Part model, mm, in its own coordinate system. A direction names the side the tool comes from. Give positions to 0.01 mm unless a question says otherwise; leave off trailing zeros. Order: outer loops, then holes, each group sorted by start corner. A loop starts at its lowest first (then second) coordinate and runs counter-clockwise, first axis right, second up.
1. Which spindle directions (+Z, -Z, +X, -X, +Y, -Y) get a long thin tool onto all of the face, cutting with end or side? Do faces 4 (the flat face through (19, -25, -8)), 5 (the cylindrical face through (4.17, 12.32, -18.8)), 6 (the flat face through (0, 25, 0)), 7 (the cylindrical face through (-15.201, -12.037, -11.655)). Say none if no direction does.
2. Drop flat-ended pins along their axis: pin 1 Ø1.5 at (y, z) = (-33, -12.5) entering from +X; pin 2 Ø8 at (x, y) = (-6.5, 8.5) entering from +Z; pin 3 Ø4 at (y, z) = (-23, 4.5) entering from -X. Give the stop position or say it passes through.
3. Mould opens along Z. For faces 1 (the cylindrical face through (20.445, -12.325, 6.438)), 2 (the flat face through (-11.2, 0, 16)), 3 (the cylindrical face through (-4.089, -12.04, -18.413)) say: +Z half, -Z half, draft (parallel to the pull), parting line (faces both ways), or undercut.
4. Slice it at C-C on y = -42.5. List the corners of the cut face in (x, z), and give its area (3 significant figures).
5. Probe line 1 (Z direction, x = 0, y = -12) (3 decimals); line 2 (X direction, y = -15, z = -1.5); line 3 (Z direction, x = 8, y = -9). List the from-to ranges inside material, lowest first.
6. Slice it at B-B on y = 14. List the corners of the cut face in (x, z), and give its area (3 significant figures).
7. Slice it at A-A on y = -11.5. List the corners of the cut face in (x, z) (3 decimals).
from build123d import *

# Parameters (mm, degrees)
F0_R     = 21.435
F0_R_2   = 19.35
F1_DEPTH = 25
F5_R     = 19.154771
F5_R_2   = 18.861777
F6_DEPTH = 25
F4_R     = 19.257792
F7_DEPTH = 25


with BuildPart() as f1:
    # F0 (on Front) → F1 (new body)
    with BuildSketch(Plane.XZ):
        Circle(F0_R)
        Circle(F0_R_2, mode=Mode.SUBTRACT)
    extrude(amount=F1_DEPTH)

    # F2 (on Right) → F3 (revolve)
    with BuildSketch(Plane.YZ):
        Polygon((-76.707862, 0), (-24.888575, 0), (-24.378041, 20.674003), align=None)
    revolve(axis=Axis((0, -6.062602, 0), (0, -1, 0)))

    # F5 (on Front) → F6 (join)
    with BuildSketch(Plane.XZ):
        Circle(F5_R)
        Circle(F5_R_2, mode=Mode.SUBTRACT)
    extrude(amount=F6_DEPTH)

    # F4 (on face) → F7 (join)
    with BuildSketch(Plane(origin=(0, 0, 0), x_dir=(-1, 0, 0), z_dir=(0, 1, 0))):
        Circle(F4_R)
    extrude(amount=F7_DEPTH)


solid = f1.part
Data:
1. face 4: -Y
1. face 5: +Y
1. face 6: +Z, -Z, +X, -X, +Y
1. face 7: none
2. pin 1: stops at x = 12.76
2. pin 2: stops at z = 19.09
2. pin 3: stops at x = -21.29
3. face 1: parting line
3. face 2: draft
3. face 3: undercut
4. outline: circle Ø27.03 at (0, 0)
4. area: 574 mm2
5. line 1: z = -21.435 to -19.35, -19.155 to -18.862, 18.862 to 19.155, 19.35 to 21.435
5. line 2: x = -21.38 to -19.29, -19.1 to -18.8, 18.8 to 19.1, 19.29 to 21.38
5. line 3: z = -19.89 to -17.62, -17.4 to -17.08, 17.08 to 17.4, 17.62 to 19.89
6. outline: circle Ø38.52 at (0, 0)
6. area: 1,170 mm2
7. outline: circle Ø42.87 at (0, 0); circle Ø38.31 at (0, 0); hole circle Ø38.7 at (0, 0); hole circle Ø37.724 at (0, 0)
